Model file for the job. Use its own axes, mm. Face numbers are marked on the shaded views. A direction names the side the tool comes from. Round coordinates to 2 decimals unless told otherwise and drop trailing zeros. Order: outer loops, then holes, each group sorted by start corner. A loop starts at its lowest first (then second) coordinate and runs counter-clockwise, first axis right, second up. Notation, with made-up numbers: (44, -2) - (99, -2) arc R23 cw to (99, 18) - close; hole circle Ø1 at (86.25, 53). An arc over 180 degrees is marked (long way). Put each result on its own line as item: value. Start each with the question number.
Item 1: Pin check, flat tips, straight feed: pin 1 Ø3 at (x, z) = (5, -0.5) entering from -Y; pin 2 Ø2 at (x, z) = (3.5, 1) entering from +Y; pin 3 Ø4 at (x, y) = (7, 1) entering from -Z. Stop position of each tip, or through.
Item 2: Which spindle directions (+Z, -Z, +X, -X, +Y, -Y) get a long thin tool onto all of the face, cutting with end or side? Do the marked faces 4, 5 and 6. Say none if no direction does.
Item 3: Saw through at A-A on x = 4. List the corners of the cut face in (y, z), plus the area to 3 significant figures.
Item 4: Mould opens along Z. For the marked faces 1, 2 and 3 say: pulls with the +Z half, pulls with the -Z half, needs draft (parallel to the pull), parting line crosses it, or undercut.
Item 5: Probe probe 1 along Y at (x, z) = (0.5, 0); probe 2 along X at (y, z) = (2.75, -0.5). List the from-to ranges inside material, lowest first.
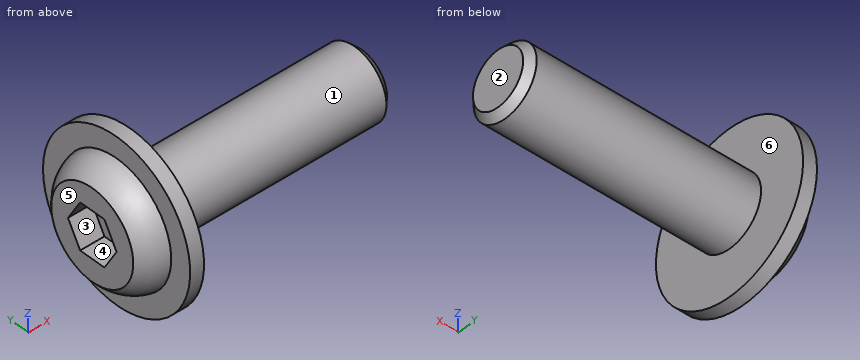
```python
from build123d import *

# Parameters (mm, degrees)
CUT_EXTRUDE1_DEPTH = 1.05


with BuildPart() as part:
    # Sketch1 → Revolve1 (revolve)
    with BuildSketch(Plane.XY):
        with BuildLine():
            Line((-1.65, 0), (-1.65, 1.95))
            ThreePointArc((-1.65, 1.95), (-1.184849394, 2.371679791), (-0.6, 2.6))
            Line((-0.6, 2.6), (-0.6, 3.5))
            Line((-0.6, 3.5), (0, 3.5))
            Line((0, 3.5), (0, 1.5))
            Line((0, 1.5), (9.6935, 1.5))
            Line((9.6935, 1.5), (10, 1.1935))
            Line((10, 1.1935), (10, 0))
            Line((10, 0), (-1.65, 0))
        make_face()
    revolve(axis=Axis((10, 0, 0), (-1, 0, 0)))

    # Sketch2 → Cut-Extrude1 (cut)
    with BuildSketch(Plane(origin=(-1.65, 0, 0), x_dir=(0, 0, -1), z_dir=(1, 0, 0))):
        Polygon((-1, -0.577350269), (0, -1.154700538), (1, -0.577350269), (1, 0.577350269), (0, 1.154700538), (-1, 0.577350269), align=None)
    extrude(amount=CUT_EXTRUDE1_DEPTH, mode=Mode.SUBTRACT)


solid = part.part
```
Results found:
1. pin 1: stops at y = -1.5
1. pin 2: stops at y = 1.5
1. pin 3: stops at z = -1.5
2. face 4: -X
2. face 5: +Z, -Z, -X, +Y, -Y
2. face 6: +X
3. outline: circle Ø3 at (0, 0)
3. area: 7.07 mm²
4. face 1: parting line crosses it
4. face 2: needs draft
4. face 3: undercut
5. probe 1: y = -1.5 to 1.5
5. probe 2: x = -0.6 to 0
